```python
from build123d import *
from build123d import SkipClean  # not in build123d's __all__

# Parameters (mm, degrees)
F1_DEPTH = 10
F2_SIZE  = 3
F3_R     = 2.821
F3_R_2   = 2.5
F4_DEPTH = 37.5
F5_DEPTH = 75


with BuildPart() as f1:
    # F0 (on Front) → F1 (new body)
    with BuildSketch(Plane.XZ):
        with BuildLine():
            ThreePointArc((37.5, 0), (26.5165042945, 26.5165042945), (0, 37.5))
            Line((0, 37.5), (0, -37.5))
            ThreePointArc((0, -37.5), (26.5165042945, -26.5165042945), (37.5, 0))
        make_face()
        with BuildLine():
            Line((0, -37.5), (0, 37.5))
            ThreePointArc((0, 37.5), (-37.5, 0), (0, -37.5))
        make_face()
    extrude(amount=F1_DEPTH)

    # F2
    f2_edges = [f1.edges().sort_by_distance(p)[0] for p in [
        (-37.5, -10, 0),
    ]]
    chamfer(f2_edges, length=F2_SIZE)

    # F3 (on Top) → F4 (join, symmetric)
    with BuildSketch(Plane.XY):
        with Locations((0, -3.2904869877)):
            Circle(F3_R)
        with Locations((0, -3.2904869877)):
            Circle(F3_R_2, mode=Mode.SUBTRACT)
    with SkipClean():  # cleaning this boolean's faces spoils the solid; the shape is the same uncleaned
        extrude(amount=F4_DEPTH, both=True)

    # F5 (add): a face of the model
    f5_faces = [f1.faces().sort_by_distance(p)[0] for p in [
        (-0.0630794776, -0.6299869877, -37.5),
    ]]
    with SkipClean():  # cleaning this boolean's faces spoils the solid; the shape is the same uncleaned
        extrude(f5_faces, amount=-F5_DEPTH)


solid = f1.part
```
Read the model definition and answer for the solid it produces. Units are mm, in the model's axes. Give positions to 0.01 mm unless a question says otherwise; leave off trailing zeros. Write each loop counter-clockwise with the first axis right and the second up, starting at its lowest first coordinate (ties: lowest second). Pieces come first, ordered by that corner, then holes. Notation, with made-up numbers: (4, 48.5) - (25, 48.5) arc R28 cw to (25, 81.5) - close; hole circle Ø2 at (31, 34.5). An arc over 180 degrees is marked (long way). Write item = value, one per line. Start each with the question number.
Item 1: Find the intervals of material crossed by probe 1 along X at (y, z) = (-1.5, 1); probe 2 along X at (y, z) = (-4, -3); probe 3 along Z at (x, y) = (-26.5, -8.5), in increasing order. Write a range as [from, to].
Item 2: Each of these flat-tipped pins is pushed along its axis until it touches: P1, Ø3, axis at x = 7.5, y = -8, coming from the +Z side; P2, Ø5, axis at x = -7.5, y = -6.5, coming from the +Z side; P3, Ø1.5, axis at x = -24, y = -2.5, coming from the +Z side. Where does it stop, or does it pass through?
Item 3: Find section A-A (y = -4.75). Give the vertices of the cut face in (x, z), then the cut area to 3 significant figures.
Response:
q1.probe_1 = [-37.49, 37.49]
q1.probe_2 = [-37.38, 37.38]
q1.probe_3 = [-24.37, 24.37]
q2.P1 = 36.95
q2.P2 = 37.17
q2.P3 = 29.42
q3.outline = (-2.41, -37.5) - (-2.03, -37.5) - (-2.03, -37.45) arc R37.5 ccw to (2.03, -37.45) - (2.03, -37.5) - (2.41, -37.5) - (2.41, -37.42) arc R37.5 ccw to (2.41, 37.42) - (2.41, 37.5) - (2.03, 37.5) - (2.03, 37.45) arc R37.5 ccw to (-2.03, 37.45) - (-2.03, 37.5) - (-2.41, 37.5) - (-2.41, 37.42) arc R37.5 ccw to (-2.41, -37.42) - close
q3.area = 4,420 mm²
